Check sheet for the modelled part. Datum: model origin and axes. Units: mm. A direction names the side the tool comes from. Round coordinates to 2 decimals unless told otherwise and drop trailing zeros. Order: outer loops, then holes, each group sorted by start corner. A loop starts at its lowest first (then second) coordinate and runs counter-clockwise, first axis right, second up. Notation, with made-up numbers: (8, -12.75) -> (12, -12.75) arc R23 cw to (12, -3.75) -> close; hole circle Ø8 at (30.25, 84). An arc over 180 degrees is marked (long way). Answer in a Markdown table with one row per item.
```python
from build123d import *

# Parameters (mm, degrees)
ESQUISSE1_W                                    = 45
ESQUISSE1_H                                    = 30
BOSS_EXTRU_1_DEPTH                             = 8
ESQUISSE5_W                                    = 30
ESQUISSE5_H                                    = 48
BOSS_EXTRU_3_DEPTH                             = 32
ENL_V_MAT_EXTRU_1_DEPTH                        = 27
ESQUISSE14_W                                   = 6
ESQUISSE14_H                                   = 8
ENL_V_MAT_EXTRU_2_DEPTH                        = 67.708320321
D_GAGEMENT_M31_D                               = 3.2
D_GAGEMENT_M31_DEPTH                           = 7
D_GAGEMENT_M31_TIP                             = 0.96137699
ESQUISSE16_W                                   = 30
ESQUISSE16_H                                   = 48
ESQUISSE16_R                                   = 3.5
BOSS_EXTRU_4_DEPTH                             = 5
CONG_1_R                                       = 2
ESQUISSE17_W                                   = 10
ESQUISSE17_H                                   = 10
ENL_V_MAT_EXTRU_3_DEPTH                        = 2
BOSS_EXTRU_5_START                             = 2
ESQUISSE18_R                                   = 6
ESQUISSE18_R_2                                 = 3.5
BOSS_EXTRU_5_DEPTH                             = 2
FRAISAGE_POUR_VIS_T_TE_FRAIS_E_M31_D           = 3.4
FRAISAGE_POUR_VIS_T_TE_FRAIS_E_M31_CSINK_D     = 6.3
FRAISAGE_POUR_VIS_T_TE_FRAIS_E_M31_CSINK_ANGLE = 90
ESQUISSE24_W                                   = 8
ESQUISSE24_H                                   = 8
BOSS_EXTRU_6_DEPTH                             = 2.6


with BuildPart() as part:
    # Esquisse1 → Boss.-Extru.1 (new body)
    with BuildSketch(Plane(origin=(0, 0, 0), x_dir=(1, 0, 0), z_dir=(0, 1, 0))):
        with Locations((10.5, 0)):
            Rectangle(ESQUISSE1_W, ESQUISSE1_H)
    extrude(amount=BOSS_EXTRU_1_DEPTH)

    # Esquisse5 → Boss.-Extru.3 (add)
    with BuildSketch(Plane.ZY.offset(12)):
        with Locations((0, 32)):
            Rectangle(ESQUISSE5_W, ESQUISSE5_H)
    extrude(amount=-BOSS_EXTRU_3_DEPTH)

    # Esquisse6 → Enl_v. mat.-Extru.1 (cut)
    with BuildSketch(Plane.ZY.offset(12)):
        Polygon((10.25, 48), (4, 48), (4, 56), (-4, 56), (-4, 48), (-10.25, 48), (-10.25, 8), (10.25, 8), align=None)
    extrude(amount=-ENL_V_MAT_EXTRU_1_DEPTH, mode=Mode.SUBTRACT)

    # Esquisse14 → Enl_v. mat.-Extru.2 (cut, through all)
    with BuildSketch(Plane(origin=(0, 56, 0), x_dir=(1, 0, 0), z_dir=(0, 1, 0))):
        with Locations((21, 0)):
            Rectangle(ESQUISSE14_W, ESQUISSE14_H)
    extrude(amount=-ENL_V_MAT_EXTRU_2_DEPTH, mode=Mode.SUBTRACT)

    # D_gagement M31
    with Locations(Plane.ZY.offset(12)):
        with Locations((5, 4), (-5, 4)):
            Hole(D_GAGEMENT_M31_D / 2, depth=D_GAGEMENT_M31_DEPTH)
            with Locations((0, 0, -(D_GAGEMENT_M31_DEPTH + D_GAGEMENT_M31_TIP / 2))):  # 118° drill point
                Cone(0, D_GAGEMENT_M31_D / 2, D_GAGEMENT_M31_TIP, mode=Mode.SUBTRACT)

    # Esquisse16 → Boss.-Extru.4 (add)
    with BuildSketch(Plane(origin=(33, 0, 0), x_dir=(0, 0, -1), z_dir=(1, 0, 0))):
        with Locations((0, 32)):
            Rectangle(ESQUISSE16_W, ESQUISSE16_H)
        with Locations((0, 38)):
            Circle(ESQUISSE16_R, mode=Mode.SUBTRACT)
    extrude(amount=-BOSS_EXTRU_4_DEPTH)

    # Cong_1
    cong_1_edges = [part.edges().sort_by_distance(p)[0] for p in [
        (24, 8, 15),
        (20, 8, -9.5),
        (20, 32, -15),
        (20, 56, 9.5),
        (4, 56, -15),
        (20, 32, 15),
        (4, 56, 15),
        (-12, 56, 9.5),
        (-12, 56, -9.5),
        (20, 8, 9.5),
        (20, 56, -9.5),
        (33, 28, 15),
        (-12, 28, 15),
        (-12, 28, -15),
        (33, 28, -15),
        (24, 8, -15),
        (28, 32, 15),
        (28, 56, 0),
        (30.5, 56, 15),
        (28, 32, -15),
        (30.5, 56, -15),
        (28, 8, 0),
        (33, 56, 0),
    ]]
    fillet(cong_1_edges, radius=CONG_1_R)

    # Esquisse17 → Enl_v. mat.-Extru.3 (cut)
    with BuildSketch(Plane.ZY.offset(-28)):
        with Locations((0, 38)):
            Rectangle(ESQUISSE17_W, ESQUISSE17_H)
    extrude(amount=-ENL_V_MAT_EXTRU_3_DEPTH, mode=Mode.SUBTRACT)

    # Esquisse18 → Boss.-Extru.5 (add)
    with BuildSketch(Plane(origin=(33, 0, 0), x_dir=(0, 0, -1), z_dir=(1, 0, 0)).offset(BOSS_EXTRU_5_START)):
        with Locations(Location((0, 38, 0), (0, 0, 180))):
            Circle(ESQUISSE18_R)
        with Locations((0, 38)):
            Circle(ESQUISSE18_R_2, mode=Mode.SUBTRACT)
    extrude(amount=-BOSS_EXTRU_5_DEPTH)

    # Fraisage pour vis _ t_te frais_e M31 (through all)
    with Locations(Plane(origin=(0, 8, 0), x_dir=(1, 0, 0), z_dir=(0, 1, 0))):
        with Locations((-7.5, 0), (7.5, 0)):
            CounterSinkHole(FRAISAGE_POUR_VIS_T_TE_FRAIS_E_M31_D / 2, FRAISAGE_POUR_VIS_T_TE_FRAIS_E_M31_CSINK_D / 2, counter_sink_angle=FRAISAGE_POUR_VIS_T_TE_FRAIS_E_M31_CSINK_ANGLE)

    # Esquisse24 → Boss.-Extru.6 (add)
    with BuildSketch(Plane.ZY.offset(-15)):
        with Locations((0, 52)):
            Rectangle(ESQUISSE24_W, ESQUISSE24_H)
    extrude(amount=BOSS_EXTRU_6_DEPTH)


solid = part.part
```
(1) Scan lines: probe 1 along Y at (x, z) = (-9, 5); probe 2 along Z at (x, y) = (-3.5, 20.5); probe 3 along Y at (x, z) = (-3, -5.5). Record each from-to range of solid material in increasing order. Write a range as from..to.
Solutions:
| item | result |
|---|---|
| probe 1 | 0..2.4, 5.6..8, 48..56 |
| probe 2 | -15..-10.25, 10.25..15 |
| probe 3 | 0..8, 48..56 |
(2) Draft check along Z on faces 6 (the cylindrical face through (20.6, 8.57, 8.56)), 7 (the cylindrical face through (-11.4, 27.38, -14.43)), 8 (the flat face through (2, 48, -5)). Enter one of: pulls with the +Z half, pulls with the -Z half, needs draft (parallel to the pull), parting line crosses it, or undercut.
Solutions:
| item | result |
|---|---|
| face 6 | needs draft |
| face 7 | pulls with the -Z half |
| face 8 | undercut |
(3) Tool access check on faces 1 (the cylindrical face through (34.014, 43.857, -1.301)), 2 (the cylindrical face through (28.57, 32.31, -14.4)), 3 (the cylindrical face through (27.43, 8.6, -0.18)), 4 (the flat face through (12.4, 52, 0)), 5 (the flat face through (30, 40.3, -3.4)). Record the directions out of +Z, -Z, +X, -X, +Y, -Y that give a thin tool (end or side, any length) a straight path to the whole face; none if there is none.
Solutions:
| item | result |
|---|---|
| face 1 | +X |
| face 2 | -Z, +Y |
| face 3 | +Z, -Z, +Y |
| face 4 | -X, +Y |
| face 5 | none |
(4) Section check B-B on y = 17. Record the boundary of the cut face in (x, z).
Solutions:
| item | result |
|---|---|
| outline | (-12, -13) arc R2 ccw to (-10, -15) -> (18, -15) arc R2 ccw to (20, -13) -> (20, -4) -> (18, -4) -> (18, 4) -> (20, 4) -> (20, 13) arc R2 ccw to (18, 15) -> (-10, 15) arc R2 ccw to (-12, 13) -> (-12, 10.25) -> (15, 10.25) -> (15, -10.25) -> (-12, -10.25) -> close; (28, -13) arc R2 ccw to (30, -15) -> (31, -15) arc R2 ccw to (33, -13) -> (33, 13) arc R2 ccw to (31, 15) -> (30, 15) arc R2 ccw to (28, 13) -> close |
(5) Section check D-D on x = 7.5. Record the boundary of the cut face in (y, z), plus the area to 3 significant figures.
Solutions:
| item | result |
|---|---|
| outline | (0, -15) -> (54, -15) arc R2 ccw to (56, -13) -> (56, -4) -> (48, -4) -> (48, -10.25) -> (8, -10.25) -> (8, -3.15) -> (6.55, -1.7) -> (0, -1.7) -> close; (0, 1.7) -> (6.55, 1.7) -> (8, 3.15) -> (8, 10.25) -> (48, 10.25) -> (48, 4) -> (56, 4) -> (56, 13) arc R2 ccw to (54, 15) -> (0, 15) -> close |
| area | 765 mm^2 |
(6) Depth check by flat-ended pin: pin 1 Ø4 at (x, z) = (-7.5, 0) entering from +Y; pin 2 Ø8 at (y, z) = (33, 2) entering from -X; pin 3 Ø1.9 at (y, z) = (4, 5) entering from -X. Enter the tip coordinate at first touch or a pass-through.
Solutions:
| item | result |
|---|---|
| pin 1 | y = 6.85 |
| pin 2 | x = 15 |
| pin 3 | x = -4.61 |
(7) Section check C-C on z = 11. Record the boundary of the cut face in (x, y).
Solutions:
| item | result |
|---|---|
| outline | (-12, 0) -> (33, 0) -> (33, 54) arc R2 ccw to (31, 56) -> (30, 56) arc R2 ccw to (28, 54) -> (28, 10) arc R2 cw to (26, 8) -> (22, 8) arc R2 cw to (20, 10) -> (20, 54) arc R2 ccw to (18, 56) -> (-10, 56) arc R2 ccw to (-12, 54) -> close |
(8) Section check A-A on x = -7.5. Record the boundary of the cut face in (y, z).
Solutions:
| item | result |
|---|---|
| outline | (0, -15) -> (54, -15) arc R2 ccw to (56, -13) -> (56, -4) -> (48, -4) -> (48, -10.25) -> (8, -10.25) -> (8, -3.15) -> (6.55, -1.7) -> (0, -1.7) -> close; (0, 1.7) -> (6.55, 1.7) -> (8, 3.15) -> (8, 10.25) -> (48, 10.25) -> (48, 4) -> (56, 4) -> (56, 13) arc R2 ccw to (54, 15) -> (0, 15) -> close; hole circle Ø3.2 at (4, -5); hole circle Ø3.2 at (4, 5) |
